from build123d import *

# Parameters (mm, degrees)
F1_DEPTH = 30
F2_R     = 5
F3_DEPTH = 30.001


with BuildPart() as f1:
    # F0 (on Right) → F1 (new body)
    with BuildSketch(Plane.YZ):
        with BuildLine():
            ThreePointArc((7.5, 52.5), (0, 60), (-7.5, 52.5))
            Line((-7.5, 52.5), (7.5, 52.5))
        make_face()
        with BuildLine():
            ThreePointArc((7.5, 52.5), (0, 45), (-7.5, 52.5))
            Line((-7.5, 52.5), (-7.5, -52.5))
            Line((-7.5, -52.5), (7.5, -52.5))
            Line((7.5, -52.5), (7.5, 52.5))
        make_face()
        with BuildLine():
            Line((7.5, 52.5), (-7.5, 52.5))
            ThreePointArc((-7.5, 52.5), (0, 45), (7.5, 52.5))
        make_face()
    extrude(amount=F1_DEPTH)

    # F2 (on face) → F3 (cut, through all)
    with BuildSketch(Plane.YZ.offset(30)):
        with Locations((0, 52.5)):
            Circle(F2_R)
    extrude(amount=-F3_DEPTH, mode=Mode.SUBTRACT)


solid = f1.part
Design review of the part built by this model. Coordinates are the model's own, in mm. Give positions to 0.01 mm unless a question says otherwise; leave off trailing zeros. Loops run counter-clockwise (first coordinate to the right, second up) from the corner with the lowest first, then second, coordinate; pieces in that order, holes last. Notation, with made-up numbers: (-4.5, 22) - (15.5, 22) arc R18 ccw to (15.5, 54) - close; hole circle Ø6 at (-5, -39). An arc over 180 degrees is marked (long way). Write item = value, one per line.
1) Clearance check with a flat-ended pin moving along its axis: pin 1 Ø1.5 at (x, y) = (16.5, 1.5) entering from +Z. State where the tip first meets the part, or that it passes through.
Result sheet:
pin_1 = 59.96
2) Take a section at B-B on x = 10.25. State the section outline as (y, z) points.
Result sheet:
outline = (-7.5, -52.5) - (7.5, -52.5) - (7.5, 52.5) arc R7.5 ccw to (-7.5, 52.5) - close; hole circle Ø10 at (0, 52.5)
3) Take a section at C-C on y = -6. State the section outline as (x, z) points, and give its area (4 significant figures).
Result sheet:
outline = (0, -52.5) - (30, -52.5) - (30, 57) - (0, 57) - close
area = 3,285 mm2
4) Take a section at A-A on y = 0. State the section outline as (x, z) points.
Result sheet:
outline = (0, -52.5) - (30, -52.5) - (30, 47.5) - (0, 47.5) - close; (0, 57.5) - (30, 57.5) - (30, 60) - (0, 60) - close
5) Draft analysis for pull direction Y (two halves, no side actions). For faces 1 (the face through (15, -7.5, 1)), 2 (the face through (15.21, -0.651, 57.457)), 3 (the face through (15, 0, 60)), state which applies: +Y half, -Y half, draft (parallel to the pull), parting line (faces both ways), or undercut.
Result sheet:
face_1 = -Y half
face_2 = undercut
face_3 = parting line
6) To check wall thickness, follow line 1 (Z direction, x = 15.75, y = 0); line 2 (Z direction, x = 18.5, y = -4); line 3 (Z direction, x = 11.5, y = -6.25). State the ranges of each line that lie inside material, in increasing order.
Result sheet:
line_1 = -52.5 to 47.5, 57.5 to 60
line_2 = -52.5 to 49.5, 55.5 to 58.84
line_3 = -52.5 to 56.65
